Geometry: final body of the model. Coordinates: model frame, mm. A direction names the side the tool comes from. Coordinates: 2 decimals unless noted, no trailing zeros. Order: outer loops, then holes, each group sorted by start corner. A loop starts at its lowest first (then second) coordinate and runs counter-clockwise, first axis right, second up. Notation, with made-up numbers: M -25,44.25 L 24,44.25 A22 ccw 24,68.25 Z; hole C -31,10 d10. An arc over 180 degrees is marked long. Use CSV: the item, a comma, the result in double quotes. Start each with the question number.
1. Section query D-D on y = -7.5. Return the cut outline in (x, z), and give its area (3 significant figures).
2. Section query A-A on x = 0. Return the cut outline in (y, z) (3 decimals).
3. First-contact query: P1, Ø2, axis at y = 4.5, z = -24, coming from the -X side; P2, Ø3, axis at y = 2.5, z = -16.5, coming from the +X side; P3, Ø4, axis at x = -2.5, z = -9.5, coming from the +Y side. Flat tips, straight axial feed; report the tip coordinate or a pass-through.
4. Material intervals for line 1 (Z direction, x = 4.5, y = 5.5); line 2 (Y direction, x = 8.5, z = -10); line 3 (Z direction, x = -2.5, y = 1), sorted ascending.
5. Set-up query: faces 4 (the flat face through (0, 0, 8)), 5 (the flat face through (3, 3, -3.5)), 6 (the flat face through (0, 1.5, 4)). Return all of +Z, -Z, +X, -X, +Y, -Y with unobstructed straight access to the full face (end or side cutting, diameter ignored); none if empty.
6. Section query C-C on z = -11.5. Return the cut outline in (x, y) (3 decimals), and give its area (3 significant figures).
7. Pull-direction query (Y, two-part tool) for faces 1 (the flat face through (-2, -2, -1.5)), 2 (the conical face through (-8.3, -0.08, -16.82)), 3 (the cylindrical face through (-3.233, -1.341, -2.486)); classes: pulls with the +Y half, pulls with the -Y half, needs draft (parallel to the pull), parting line crosses it, or undercut.
8. Section query B-B on z = -21. Return the cut outline in (x, y) (3 decimals).
from build123d import *

# Parameters (mm, degrees)
BOSS_EXTRUDE1_DEPTH   = 8
BOSS_EXTRUDE2_START   = 1.5
SKETCH2_R             = 2
BOSS_EXTRUDE2_DEPTH   = 1.5
SKETCH3_R             = 3.5
BOSS_EXTRUDE3_DEPTH   = 2
SKETCH4_R             = 12.425
BOSS_EXTRUDE4_DEPTH   = 51.8
M3_TAPPED_HOLE1_D     = 2.5
M3_TAPPED_HOLE1_DEPTH = 12.7
M3_TAPPED_HOLE1_TIP   = 0.751075774


with BuildPart() as part:
    # Sketch1 → Boss-Extrude1 (new body)
    with BuildSketch(Plane.XY):
        with BuildLine():
            Line((-1.322875656, 1.5), (1.322875656, 1.5))
            ThreePointArc((1.322875656, 1.5), (0, -2), (-1.322875656, 1.5))
        make_face()
    extrude(amount=BOSS_EXTRUDE1_DEPTH)

    # Sketch2 → Boss-Extrude2 (add)
    with BuildSketch(Plane(origin=(0, 0, 0), x_dir=(-1, 0, 0), z_dir=(0, 0, -1)).offset(BOSS_EXTRUDE2_START)):
        Circle(SKETCH2_R)
    extrude(amount=-BOSS_EXTRUDE2_DEPTH)

    # Sketch3 → Boss-Extrude3 (add)
    with BuildSketch(Plane(origin=(0, 0, -1.5), x_dir=(-1, 0, 0), z_dir=(0, 0, -1))):
        Circle(SKETCH3_R)
    extrude(amount=BOSS_EXTRUDE3_DEPTH)

    # Sketch4 → Boss-Extrude4 (add)
    with BuildSketch(Plane(origin=(0, 0, -3.5), x_dir=(-1, 0, 0), z_dir=(0, 0, -1))):
        with Locations(Location((0, 0, 0), (0, 0, 180))):
            Circle(SKETCH4_R)
    extrude(amount=BOSS_EXTRUDE4_DEPTH)

    # M3 Tapped Hole1
    with Locations(Plane.XY.offset(-3.5)):
        with Locations((8.5, 0), (-8.5, 0)):
            Hole(M3_TAPPED_HOLE1_D / 2, depth=M3_TAPPED_HOLE1_DEPTH)
            with Locations((0, 0, -(M3_TAPPED_HOLE1_DEPTH + M3_TAPPED_HOLE1_TIP / 2))):  # 118° drill point
                Cone(0, M3_TAPPED_HOLE1_D / 2, M3_TAPPED_HOLE1_TIP, mode=Mode.SUBTRACT)


solid = part.part
Results list:
1,outline,"M -9.91,-55.3 L 9.91,-55.3 L 9.91,-3.5 L -9.91,-3.5 Z"
1,area,"1,030 mm²"
2,outline,"M -12.425,-55.3 L 12.425,-55.3 L 12.425,-3.5 L 3.5,-3.5 L 3.5,-1.5 L 2,-1.5 L 2,0 L 1.5,0 L 1.5,8 L -2,8 L -2,-1.5 L -3.5,-1.5 L -3.5,-3.5 L -12.425,-3.5 Z"
3,P1,"stops at x = -11.92"
3,P2,"stops at x = 12.38"
3,P3,"stops at y = 12.41"
4,line 1,"z = -55.3 to -3.5"
4,line 2,"y = -9.06 to -1.25, 1.25 to 9.06"
4,line 3,"z = -55.3 to -1.5"
5,face 4,"+Z, +X, -X, +Y, -Y"
5,face 5,"+Z"
5,face 6,"+Z, +X, -X, +Y"
6,outline,"C 0,0 d24.85; hole C -8.5,0 d2.5; hole C 8.5,0 d2.5"
6,area,"475 mm²"
7,face 1,"needs draft"
7,face 2,"undercut"
7,face 3,"parting line crosses it"
8,outline,"C 0,0 d24.85"
